Work out the finished part from the listing and answer in its coordinate system (mm). Face numbers are marked on the shaded views. Coordinates: 2 decimals unless noted, no trailing zeros. Order: outer loops, then holes, each group sorted by start corner. A loop starts at its lowest first (then second) coordinate and runs counter-clockwise, first axis right, second up. Notation, with made-up numbers: (22.5, -37) -> (35.5, -37) arc R27 cw to (35.5, -5) -> close; hole circle Ø4 at (5.25, -25.5). An arc over 180 degrees is marked (long way). Write item = value, one per line. Start each with the question number.
Q1. Flat-ended cylindrical pins translate along their axes: pin 1 (10 mm diameter, centred on y = -9.5, z = 17, fed in from +X); pin 2 (1 mm diameter, centred on x = -26.5, z = -12.5, fed in from -Y); pin 3 (6 mm diameter, centred on x = -5.5, z = -11, fed in from -Y); pin 4 (4.5 mm diameter, centred on x = -13, y = -13.5, fed in from -Z). Find the tip coordinate at first contact, or state that the pin passes through.
Q2. The part is cut by section D-D, the plane y = -7.25. Determine the outline of the cut face in (x, z) (1 decimal), plus the area to 3 significant figures.
Q3. The part is cut by section A-A, the plane x = 0. Determine the outline of the cut face in (y, z).
Q4. The part is cut by section B-B, the plane y = -14. Determine the outline of the cut face in (x, z) (1 decimal), plus the area to 3 significant figures.
Q5. The part is cut by section C-C, the plane z = 0. Determine the outline of the cut face in (x, y), plus the area to 3 significant figures.
Q6. For a pull along Z with two mould halves and no side action, classify the marked faces 1, 2 and 3 as +Z half, -Z half, draft (parallel to the pull), parting line (faces both ways), or undercut.
Q7. Straight lines are drawn through the part: L1, parallel to Z at x = 0, y = -23; L2, parallel to Z at x = 0, y = -0.75; L3, parallel to Z at x = 6, y = -16.25. For each, find the intervals that lie inside material, in ascending order. Write a range as from..to.
```python
from build123d import *

# Parameters (mm, degrees)
F0_R      = 30.1625
F1_DEPTH  = 15.24
F2_D      = 2.54
F3_DEPTH  = 10.922
F4_D      = 1.27
F5_R      = 34.2265
F5_R_2    = 30.1625
F6_DEPTH  = 25.4
F8_W      = 6.35
F8_H      = 2.54
F8_H_2    = 6.35
F9_DEPTH  = 8.382
F10_D     = 2.54
F10_DEPTH = 10.161
F0_W      = 76.2
F0_H      = 76.2
F11_DEPTH = 2.54
F12_D     = 2.54
F13_W     = 76.2
F13_H     = 76.2
F13_R     = 11.0948644811
F14_DEPTH = 1.27
F15_D     = 2.54


with BuildPart() as f1:
    # F0 (on Front) → F1 (new body)
    with BuildSketch(Plane.XZ):
        Circle(F0_R)
        with BuildLine():
            ThreePointArc((-11.329190163, -11.811), (0, -2.9845), (11.329190163, -11.811))
            Line((11.329190163, -11.811), (15.875, -11.811))
            ThreePointArc((15.875, -11.811), (17.8955576272, -12.6479423728), (18.7325, -14.6685))
            ThreePointArc((18.7325, -14.6685), (17.8955576272, -16.6890576272), (15.875, -17.526))
            Line((15.875, -17.526), (11.329190163, -17.526))
            ThreePointArc((11.329190163, -17.526), (0, -26.3525), (-11.329190163, -17.526))
            Line((-11.329190163, -17.526), (-15.875, -17.526))
            ThreePointArc((-15.875, -17.526), (-18.7325, -14.6685), (-15.875, -11.811))
            Line((-15.875, -11.811), (-11.329190163, -11.811))
        make_face(mode=Mode.SUBTRACT)
    extrude(amount=F1_DEPTH)

    # F2 (through all)
    with Locations(Plane(origin=(0, 0, 0), x_dir=(1, 0, 0), z_dir=(0, 1, 0))):
        with Locations((-10.414, 19.3421), (10.414, 19.3421)):
            Hole(F2_D / 2)

    # F0 (on Front) → F3 (join)
    with BuildSketch(Plane.XZ):
        with BuildLine():
            ThreePointArc((-13.0175, -14.6685), (-13.8544423728, -12.6479423728), (-15.875, -11.811))
            Line((-15.875, -11.811), (-15.875, -17.526))
            ThreePointArc((-15.875, -17.526), (-13.8544423728, -16.6890576272), (-13.0175, -14.6685))
        make_face()
        with BuildLine():
            Line((-15.875, -17.526), (-15.875, -11.811))
            ThreePointArc((-15.875, -11.811), (-18.7325, -14.6685), (-15.875, -17.526))
        make_face()
        with BuildLine():
            Line((15.875, -17.526), (15.875, -11.811))
            ThreePointArc((15.875, -11.811), (13.0175, -14.6685), (15.875, -17.526))
        make_face()
        with BuildLine():
            ThreePointArc((18.7325, -14.6685), (17.8955576272, -12.6479423728), (15.875, -11.811))
            Line((15.875, -11.811), (15.875, -17.526))
            ThreePointArc((15.875, -17.526), (17.8955576272, -16.6890576272), (18.7325, -14.6685))
        make_face()
        with BuildLine():
            ThreePointArc((-11.329190163, -17.526), (-11.684, -14.6685), (-11.329190163, -11.811))
            Line((-11.329190163, -11.811), (-15.875, -11.811))
            ThreePointArc((-15.875, -11.811), (-13.8544423728, -12.6479423728), (-13.0175, -14.6685))
            ThreePointArc((-13.0175, -14.6685), (-13.8544423728, -16.6890576272), (-15.875, -17.526))
            Line((-15.875, -17.526), (-11.329190163, -17.526))
        make_face()
        with BuildLine():
            ThreePointArc((11.329190163, -11.811), (11.5949582549, -13.2287781284), (11.684, -14.6685))
            ThreePointArc((11.684, -14.6685), (11.5949582549, -16.1082218716), (11.329190163, -17.526))
            Line((11.329190163, -17.526), (15.875, -17.526))
            ThreePointArc((15.875, -17.526), (13.0175, -14.6685), (15.875, -11.811))
            Line((15.875, -11.811), (11.329190163, -11.811))
        make_face()
    extrude(amount=F3_DEPTH)

    # F4 (through all)
    with Locations(Plane(origin=(0, 0, 0), x_dir=(1, 0, 0), z_dir=(0, 1, 0))):
        with Locations((-15.875, 14.6685), (15.875, 14.6685)):
            Hole(F4_D / 2)

    # F5 (on Front) → F6 (join)
    with BuildSketch(Plane.XZ):
        Circle(F5_R)
        Circle(F5_R_2, mode=Mode.SUBTRACT)
    extrude(amount=F6_DEPTH)

    # F8 (on offset) → F9 (join)
    with BuildSketch(Plane.XZ.offset(15.24)):
        with Locations((0, -28.2834693789)):
            Rectangle(F8_W, F8_H)
        with Locations((-21.209, -6.1595)):
            Rectangle(F8_W, F8_H_2)
        with Locations((21.209, -6.1595)):
            Rectangle(F8_W, F8_H_2)
    extrude(amount=F9_DEPTH)

    # F10 (through all, one way)
    with BuildSketch(Plane(origin=(0, -15.24, 0), x_dir=(1, 0, 0), z_dir=(0, 1, 0))):
        with Locations((-21.209, 6.1595), (21.209, 6.1595)):
            Circle(F10_D / 2)
    extrude(amount=-F10_DEPTH, mode=Mode.SUBTRACT)

    # F0 (on Front) → F11 (join)
    with BuildSketch(Plane.XZ):
        Rectangle(F0_W, F0_H)
        Circle(F0_R, mode=Mode.SUBTRACT)
    extrude(amount=F11_DEPTH)

    # F12 (through all)
    with Locations(Plane(origin=(0, 0, 0), x_dir=(1, 0, 0), z_dir=(0, 1, 0))):
        with Locations((31.5595, 31.5595), (-31.5595, 31.5595), (-31.5595, -31.5595), (31.5595, -31.5595)):
            Hole(F12_D / 2)

    # F13 (on Front) → F14 (join)
    with BuildSketch(Plane.XZ):
        Rectangle(F13_W, F13_H)
        with Locations((0, -14.6812)):
            Circle(F13_R, mode=Mode.SUBTRACT)
    extrude(amount=F14_DEPTH)

    # F15 (through all)
    with Locations(Plane(origin=(0, 0, 0), x_dir=(1, 0, 0), z_dir=(0, 1, 0))):
        with Locations((10.414, 19.3548), (-10.414, 19.3548)):
            Hole(F15_D / 2)


solid = f1.part
```
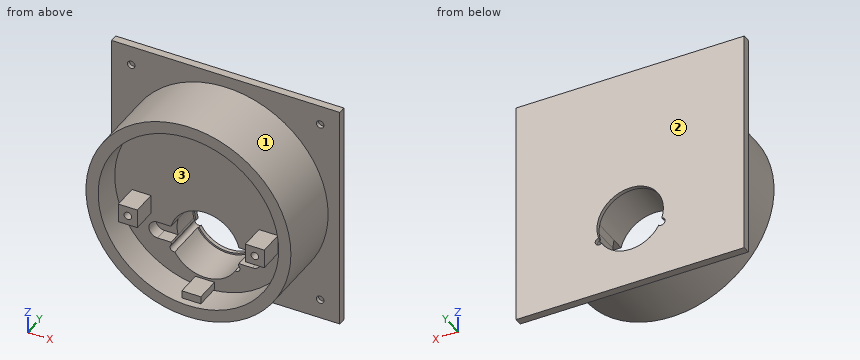
Model answer:
q1.pin_1 = 32.05
q1.pin_2 = -15.24
q1.pin_3 = through
q1.pin_4 = -32.49
q2.outline = circle Ø68.5 at (0, 0); hole circle Ø1.3 at (-15.9, -14.7); hole (-11.7, -19.3) arc R1.3 ccw to (-10.1, -20.6) arc R11.7 ccw to (10.1, -20.6) arc R1.3 ccw to (11.7, -19.3) arc R1.3 ccw to (11.1, -18.3) arc R11.7 ccw (long way) to (-11.1, -18.3) arc R1.3 ccw to start; hole circle Ø1.3 at (15.9, -14.7)
q2.area = 3,240 mm2
q3.outline = (-25.4, -34.23) -> (-2.54, -34.23) -> (-2.54, -38.1) -> (0, -38.1) -> (0, -25.78) -> (-1.27, -25.78) -> (-1.27, -26.35) -> (-15.24, -26.35) -> (-15.24, -27.01) -> (-23.62, -27.01) -> (-23.62, -29.55) -> (-15.24, -29.55) -> (-15.24, -30.16) -> (-25.4, -30.16) -> close; (-25.4, 30.16) -> (-15.24, 30.16) -> (-15.24, -2.98) -> (-1.27, -2.98) -> (-1.27, -3.59) -> (0, -3.59) -> (0, 38.1) -> (-2.54, 38.1) -> (-2.54, 34.23) -> (-25.4, 34.23) -> close
q4.outline = circle Ø68.5 at (0, 0); hole (-15.9, -17.5) -> (-11.3, -17.5) arc R11.7 ccw to (-11.1, -18.3) arc R1.3 ccw to (-11.7, -19.3) arc R1.3 ccw to (-10.1, -20.6) arc R11.7 ccw to (10.1, -20.6) arc R1.3 ccw to (11.7, -19.3) arc R1.3 ccw to (11.1, -18.3) arc R11.7 ccw to (11.3, -17.5) -> (15.9, -17.5) arc R2.9 ccw to (15.9, -11.8) -> (11.3, -11.8) arc R11.7 ccw to (-11.3, -11.8) -> (-15.9, -11.8) arc R2.9 ccw to start
q4.area = 3,170 mm2
q5.outline = (-38.1, -2.54) -> (-34.23, -2.54) -> (-34.23, -25.4) -> (-30.16, -25.4) -> (-30.16, -15.24) -> (30.16, -15.24) -> (30.16, -25.4) -> (34.23, -25.4) -> (34.23, -2.54) -> (38.1, -2.54) -> (38.1, 0) -> (-38.1, 0) -> close
q5.area = 1,150 mm2
q6.face_1 = parting line
q6.face_2 = draft
q6.face_3 = undercut
q7.L1 = -34.23..-30.16, -29.55..-27.01, 30.16..34.23
q7.L2 = -38.1..-25.78, -3.59..38.1
q7.L3 = -33.7..-29.56, 29.56..33.7
